Geometry: see drawing. Coordinates: mm, zero at the bounding-box minimum. A direction names the side the tool comes from. Coordinates: 2 decimals unless noted, no trailing zeros. Loops run counter-clockwise (first coordinate to the right, second up) from the corner with the lowest first, then second, coordinate; pieces in that order, holes last. Notation, with made-up numbers: (32.25, 66.5) - (81.25, 66.5) arc R31 ccw to (81.25, 96.5) - close; hole circle Ø4 at (-19.75, 72.5). An arc over 180 degrees is marked (long way). Use a Markdown table: item, result. Add a question column.
1. Draft query along Z for the marked faces 3, 4, 5 and 6. Return one class per face: released by +Z, released by -Z, zero draft, split by the parting line, or undercut.
2. Access query for the marked faces 1 and 2. Directions: +Z, -Z, +X, -X, +Y, -Y. A direction counts if a zero-diameter tool reaches every point of the face in a straight line with its end or side. Return the directions, or none.
3. Ray query, L1, parallel to Z at x = 15.25, y = 9.5; L2, parallel to Y at x = 8, z = 4.75; L3, parallel to Y at x = 14, z = 9.5. Return the intervals inside material, ascending. Write a range as [from, to].
4. Section query C-C on z = 13.5. Return the cut outline in (x, y), then the cut area to 3 significant figures.
5. Contact query for flat-ended pins moving along their axis: P1, Ø1.5, axis at y = 12, z = 8.5, coming from the +X side; P2, Ø5, axis at x = 12, z = 12.5, coming from the -Y side; P3, Ø1.5, axis at y = 2, z = 6.5, coming from the -X side. Output: stop coordinate, or through.
6. Section query D-D on y = 3.75. Return the cut outline in (x, z), then the cut area to 3 significant figures.
7. Section query A-A on x = 8. Return the cut outline in (y, z).
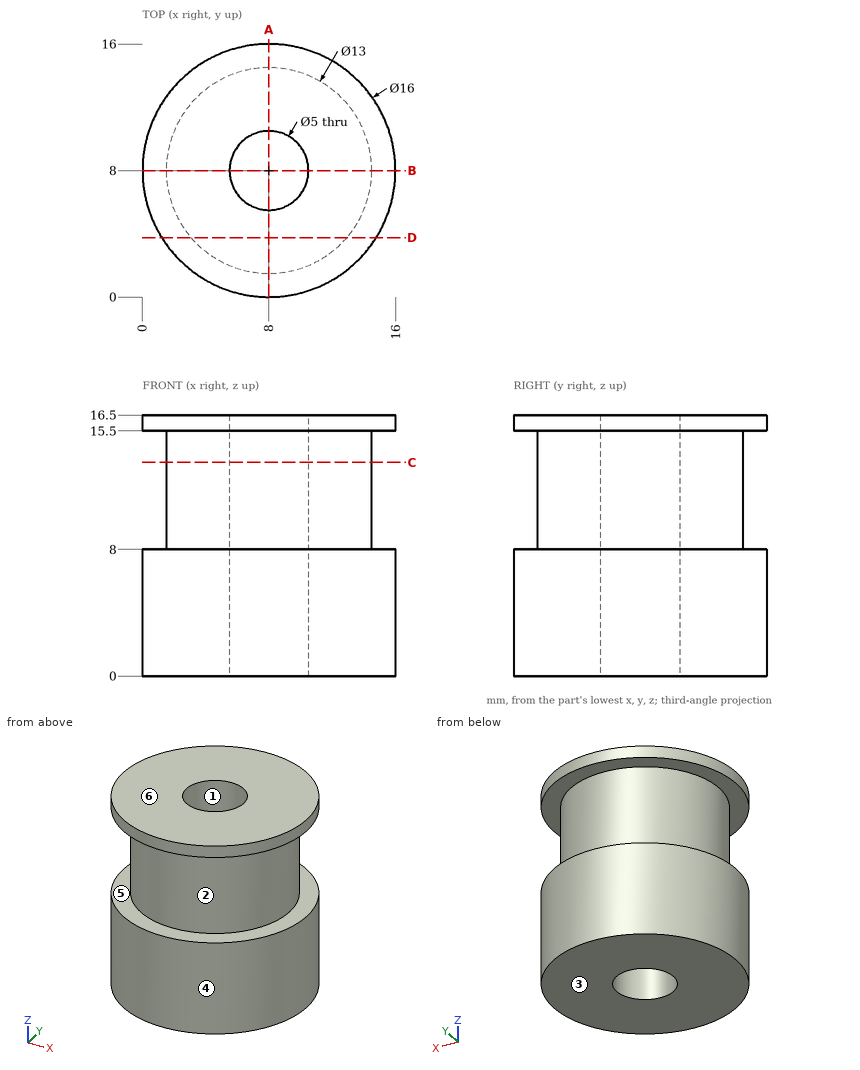
Resolved:
| question | item | result |
|---|---|---|
| 1 | face 3 | released by -Z |
| 1 | face 4 | zero draft |
| 1 | face 5 | undercut |
| 1 | face 6 | released by +Z |
| 2 | face 1 | +Z, -Z |
| 2 | face 2 | none |
| 3 | L1 | [0, 8], [15.5, 16.5] |
| 3 | L2 | [0, 5.5], [10.5, 16] |
| 3 | L3 | [5.5, 10.5] |
| 4 | outline | circle Ø13 at (8, 8); hole circle Ø5 at (8, 8) |
| 4 | area | 113 mm² |
| 5 | P1 | x = 15.22 |
| 5 | P2 | y = 1.68 |
| 5 | P3 | x = 1.96 |
| 6 | outline | (1.22, 0) - (14.78, 0) - (14.78, 8) - (12.92, 8) - (12.92, 15.5) - (14.78, 15.5) - (14.78, 16.5) - (1.22, 16.5) - (1.22, 15.5) - (3.08, 15.5) - (3.08, 8) - (1.22, 8) - close |
| 6 | area | 196 mm² |
| 7 | outline | (0, 0) - (5.5, 0) - (5.5, 16.5) - (0, 16.5) - (0, 15.5) - (1.5, 15.5) - (1.5, 8) - (0, 8) - close; (10.5, 0) - (16, 0) - (16, 8) - (14.5, 8) - (14.5, 15.5) - (16, 15.5) - (16, 16.5) - (10.5, 16.5) - close |
